Geometry check sheet. Reference: drawing and pictorial views, mm from the part's lowest x, y, z. Round coordinates to 2 decimals unless told otherwise and drop trailing zeros. Loops run counter-clockwise (first coordinate to the right, second up) from the corner with the lowest first, then second, coordinate; pieces in that order, holes last. Notation, with made-up numbers: (36.25, 86) - (77.25, 86) arc R20 cw to (77.25, 112) - close; hole circle Ø9 at (8, 37.25). An arc over 180 degrees is marked (long way). Put each result on its own line as item: value. Start each with the question number.
Item 1: Gauge pin test, flat ends, axial feed: pin 1 Ø5 at (x, y) = (25, 28) entering from -Z; pin 2 Ø3 at (y, z) = (6, 57.5) entering from +X; pin 3 Ø11 at (y, z) = (4, 53) entering from -X. Record the tip position at first contact, or that the pin passes through.
Item 2: Material ranges on line 1 along X through (y, z) = (3, 40); line 2 along Y through (x, z) = (112, 8.5); line 3 along Z through (x, y) = (25, 45.5), recorded low to high.
Item 3: Section check D-D, the plane z = 61.5. Record the cut outline in (x, y), and give its area (3 significant figures).
Item 4: Draft check along Y on the marked faces 1, 2 and 3. Enter one of: pulls with the +Y half, pulls with the -Y half, needs draft (parallel to the pull), parting line crosses it, or undercut.
Item 5: Section check C-C, the plane z = 46.5. Record the cut outline in (x, y).
Item 6: Section check A-A, the plane y = 8. Record the cut outline in (x, z).
Item 7: Section check B-B, the plane x = 90. Record the cut outline in (y, z), and give its area (3 significant figures).
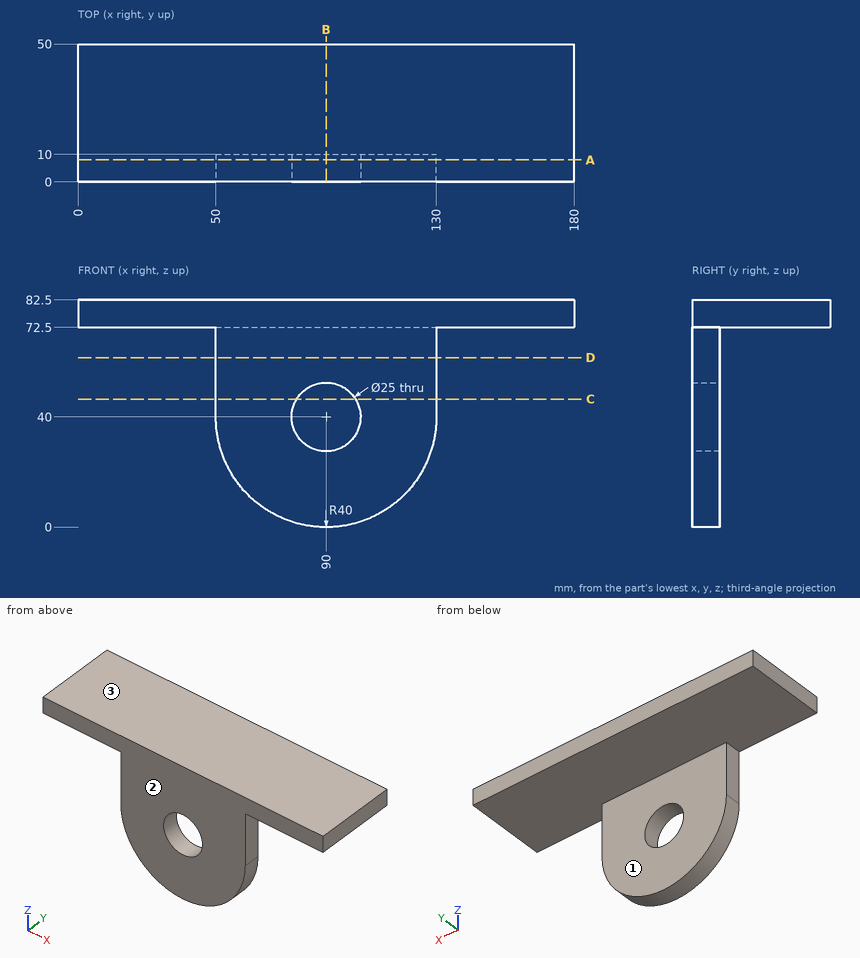
Check result:
1. pin 1: z = 72.5
1. pin 2: x = 130
1. pin 3: x = 50
2. line 1: 50 to 77.5, 102.5 to 130
2. line 2: 0 to 10
2. line 3: 72.5 to 82.5
3. outline: (50, 0) - (130, 0) - (130, 10) - (50, 10) - close
3. area: 800 mm²
4. face 1: pulls with the +Y half
4. face 2: pulls with the -Y half
4. face 3: needs draft
5. outline: (50, 0) - (79.32, 0) - (79.32, 10) - (50, 10) - close; (100.68, 0) - (130, 0) - (130, 10) - (100.68, 10) - close
6. outline: (0, 72.5) - (50, 72.5) - (50, 40) arc R40 ccw to (130, 40) - (130, 72.5) - (180, 72.5) - (180, 82.5) - (0, 82.5) - close; hole circle Ø25 at (90, 40)
7. outline: (0, 0) - (10, 0) - (10, 27.5) - (0, 27.5) - close; (0, 52.5) - (10, 52.5) - (10, 72.5) - (50, 72.5) - (50, 82.5) - (0, 82.5) - close
7. area: 975 mm²
